Part model, mm, in its own coordinate system. A direction names the side the tool comes from. Round coordinates to 2 decimals unless told otherwise and drop trailing zeros. Write each loop counter-clockwise with the first axis right and the second up, starting at its lowest first coordinate (ties: lowest second). Pieces come first, ordered by that corner, then holes.
1) Which spindle directions (+Z, -Z, +X, -X, +Y, -Y) get a long thin tool onto all of the face, cutting with end or side? Do faces 1 (the flat face through (-1, 6, -32)), 2 (the cylindrical face through (2.27, 8.86, -38.59)). Say none if no direction does.
2) Drill centre lines: L1, parallel to X at y = 7.5, z = -37; L2, parallel to X at y = 3.25, z = 0; L3, parallel to Z at x = -2, y = 6.75. Where is each one in solid material? Low to high.
3) Saw through at C-C on y = 5. Write the cut outline in (x, z).
4) Saw through at B-B on z = 0. Write the cut outline in (x, y).
5) Flat gauge pins, fed straight in: pin 1 (3 mm diameter, centred on y = 3.5, z = -32.5, fed in from -X); pin 2 (2 mm diameter, centred on y = 2, z = 21.5, fed in from +X); pin 3 (5 mm diameter, centred on x = 12.5, y = 5, fed in from -Z). Where does each tip first touch, or does it go through?
6) Pull direction X, two halves, no side cores. Call faces 3 (the flat face through (3.5, 3, -33)), 4 (the flat face through (1, 5, -32)), 5 (the cylindrical face through (-2.23, 8.8, -38.65)), 6 (the flat face through (-3.5, 3, -33)): +X half, -X half, draft (parallel to the pull), parting line (faces both ways), or undercut.
7) Saw through at D-D on x = 5. Write the cut outline in (y, z).
8) Saw through at A-A on x = -2.5. Write the cut outline in (y, z), and give its area (3 significant figures).
```python
from build123d import *

# Parameters (mm, degrees)
SALIENTE_EXTRUIR1_DEPTH = 10
CROQUIS3_R              = 2.5
CORTAR_EXTRUIR1_DEPTH   = 10
REDONDEO1_R             = 4


with BuildPart() as part:
    # Croquis2 → Saliente-Extruir1 (new body)
    with BuildSketch(Plane(origin=(0, 0, 0), x_dir=(1, 0, 0), z_dir=(0, 1, 0))):
        with BuildLine():
            Line((-1, 39.795133831), (-1, 27.481812167))
            ThreePointArc((-1, 27.481812167), (0, -27.5), (1, 27.481812167))
            Line((1, 27.481812167), (1, 39.795133831))
            Line((1, 39.795133831), (3.5, 39.795133831))
            Line((3.5, 39.795133831), (3.5, 29.795133831))
            ThreePointArc((3.5, 29.795133831), (0, -30), (-3.5, 29.795133831))
            Line((-3.5, 29.795133831), (-3.5, 39.795133831))
            Line((-3.5, 39.795133831), (-1, 39.795133831))
        make_face()
    extrude(amount=SALIENTE_EXTRUIR1_DEPTH)

    # Croquis3 → Cortar-Extruir1 (cut)
    with BuildSketch(Plane.ZY.offset(3.5)):
        with Locations((-34.795133831, 5)):
            Circle(CROQUIS3_R)
    extrude(amount=-CORTAR_EXTRUIR1_DEPTH, mode=Mode.SUBTRACT)

    # Redondeo1
    redondeo1_edges = [part.edges().sort_by_distance(p)[0] for p in [
        (-2.25, 0, -39.795133831),
        (-2.25, 10, -39.795133831),
        (2.25, 10, -39.795133831),
        (2.25, 0, -39.795133831),
    ]]
    fillet(redondeo1_edges, radius=REDONDEO1_R)


solid = part.part
```
Completed:
1. face 1: -Z, +Y, -Y
1. face 2: -Z, +X, -X, +Y
2. L1: x = -3.5 to -1, 1 to 3.5
2. L2: x = -30 to -27.5, 27.5 to 30
2. L3: z = -39.72 to -36.58, -33.01 to -27.43, 27.43 to 29.93
3. outline: (-3.5, -39.8) - (-1, -39.8) - (-1, -37.3) - (-3.5, -37.3) - close; (-3.5, -32.3) - (-1, -32.3) - (-1, -27.48) arc R27.5 cw (long way) to (1, -27.48) - (1, -32.3) - (3.5, -32.3) - (3.5, -29.8) arc R30 ccw (long way) to (-3.5, -29.8) - close; (1, -39.8) - (3.5, -39.8) - (3.5, -37.3) - (1, -37.3) - close
4. outline: (-30, 0) - (-27.5, 0) - (-27.5, 10) - (-30, 10) - close; (27.5, 0) - (30, 0) - (30, 10) - (27.5, 10) - close
5. pin 1: stops at x = -3.5
5. pin 2: stops at x = 21.9
5. pin 3: stops at z = -28.28
6. face 3: +X half
6. face 4: undercut
6. face 5: draft
6. face 6: -X half
7. outline: (0, -29.58) - (10, -29.58) - (10, -27.04) - (0, -27.04) - close; (0, 27.04) - (10, 27.04) - (10, 29.58) - (0, 29.58) - close
8. outline: (0, -35.8) arc R4 ccw to (4, -39.8) - (6, -39.8) arc R4 ccw to (10, -35.8) - (10, -27.39) - (0, -27.39) - close; (0, 27.39) - (10, 27.39) - (10, 29.9) - (0, 29.9) - close; hole circle Ø5 at (5, -34.8)
8. area: 123 mm2
